For this review, use the dimensioned drawing (mm, ordinates from the lowest corner) and the shaded views. A direction names the side the tool comes from. Give positions to 0.01 mm unless a question says otherwise; leave off trailing zeros. Write each loop counter-clockwise with the first axis right and the second up, starting at its lowest first coordinate (ties: lowest second). Pieces come first, ordered by that corner, then holes. Notation, with made-up numbers: M -16,-38 L 25,-38 A10 cw 25,-26 Z; hole C 16.25,54.5 d11. An arc over 180 degrees is marked long. One line per item, written item: value. Start each with the question number.
Item 1: Consider section D-D, the plane x = 5.5. Write out the cut boundary in (y, z).
Item 2: Consider section A-A, the plane x = 10. Write out the cut boundary in (y, z), and give its area (3 significant figures).
Item 3: Clearance check with flat-ended pins moving along their axes: pin 1 Ø1.5 at (x, z) = (8, 3.5) entering from -Y; pin 2 Ø4 at (x, y) = (4, 12) entering from -Z; pin 3 Ø3 at (x, z) = (3, 6) entering from +Y. State where each tip first meets the part, or that it passes through.
Item 4: To check wall thickness, follow probe 1 along X at (y, z) = (12.25, 7.5); probe 2 along X at (y, z) = (8.5, 4); probe 3 along Y at (x, z) = (11, 1.5). State the ranges of each line that lie inside material, in increasing order.
Item 5: Mouldability with a two-part tool opening along Y and no side actions: class the marked faces 3, 4 and 5 as released by +Y, released by -Y, zero draft, split by the parting line, or undercut.
Item 6: Consider section B-B, the plane y = 10. Write out the cut boundary in (x, z), and give its area (4 significant figures).
Item 7: Tool access review of the marked faces 1 and 2: name each direction out of +Z, -Z, +X, -X, +Y, -Y from which nothing blocks a thin tool from reaching the whole face with its end or side.
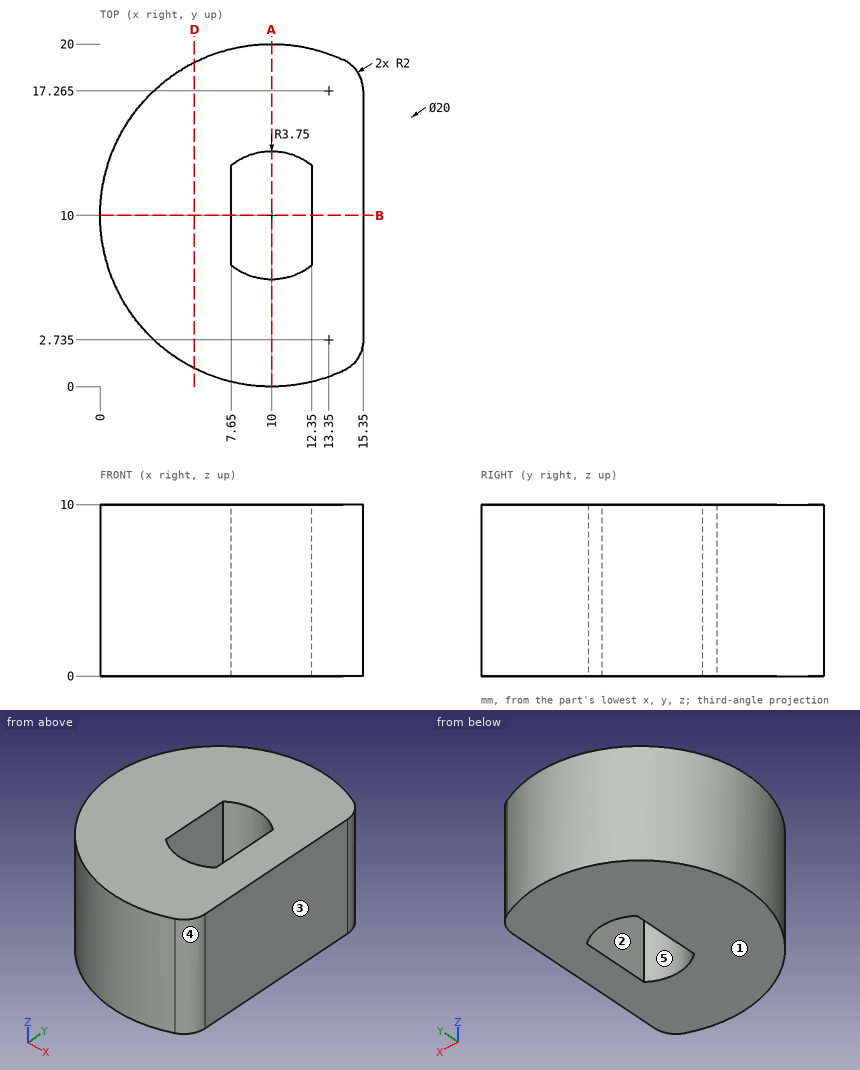
Model answer:
1. outline: M 1.07,0 L 18.93,0 L 18.93,10 L 1.07,10 Z
2. outline: M 0,0 L 6.25,0 L 6.25,10 L 0,10 Z; M 13.75,0 L 20,0 L 20,10 L 13.75,10 Z
2. area: 125 mm2
3. pin 1: stops at y = 0.08
3. pin 2: stops at z = 0
3. pin 3: stops at y = 18.35
4. probe 1: x = 0.26 to 7.65, 12.35 to 15.35
4. probe 2: x = 0.11 to 7.65, 12.35 to 15.35
4. probe 3: y = 0.05 to 6.39, 13.61 to 19.95
5. face 3: zero draft
5. face 4: released by -Y
5. face 5: undercut
6. outline: M 0,0 L 7.65,0 L 7.65,10 L 0,10 Z; M 12.35,0 L 15.35,0 L 15.35,10 L 12.35,10 Z
6. area: 106.5 mm2
7. face 1: -Z, +X, -X, +Y, -Y
7. face 2: +Z, -Z
